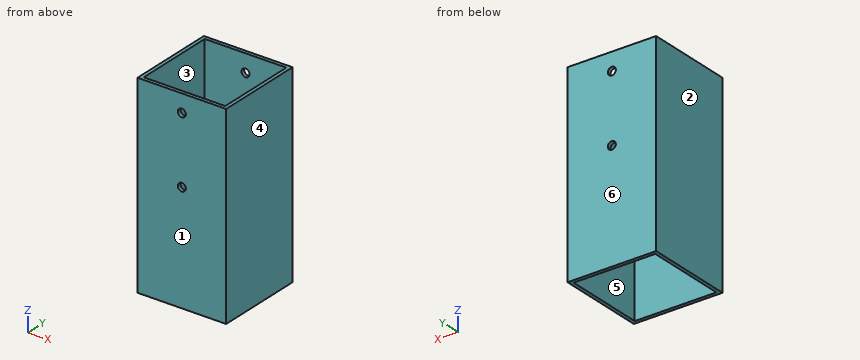
Autodesk Inventor part; units mm, degrees
ref_plane "YZ Plane" through (0, 0, 0) normal (1, 0, 0) x (0, 1, 0)
ref_plane "XZ Plane" through (0, 0, 0) normal (0, 1, 0) x (-1, 0, 0)
ref_plane "XY Plane" through (0, 0, 0) normal (0, 0, 1) x (1, 0, 0)
sketch "スケッチ1" plane through (0, 0, 0) normal (0, 0, 1) x (1, 0, 0)
  line L0 (0, 0) -> (50, 0)
  line L1 (50, 0) -> (50, 50)
  line L2 (50, 50) -> (0, 50)
  line L3 (0, 50) -> (0, 0)
  line L4 (2, 48) -> (48, 48)
  line L5 (48, 48) -> (48, 2)
  line L6 (48, 2) -> (2, 2)
  line L7 (2, 2) -> (2, 48)
  dimension "d0" = 50
  dimension "d1" = 50
  dimension "d2" = 2
extrude "押し出し1" add sketch "スケッチ1" along normal blind 110
sketch "スケッチ5" plane through (0, 50, 0) normal (0, 1, 0) x (1, 0, 0)
  line L0 (50, 0) -> (0, 0)
  line L1 (0, 0) -> (0, -110)
  line L2 (50, -110) -> (0, -110)
  line L3 (50, 0) -> (50, -110)
  line L4 (25, 0) -> (25, -110) construction
  point P0 (0, 0)
  point P1 (25, -62)
  point P2 (25, -100)
  dimension "d42" = 38
  dimension "d43" = 10
hole "穴4" at (25, 50, 62) at (25, 50, 100) direction (0, -1, 0) diameter 4.5 end through all
properties part number "center" material "アルミニウム 6061"
Read the model definition and answer for the solid it produces. Units are mm, in the model's axes. Face numbers are marked on the shaded views. A direction names the side the tool comes from. Coordinates: 2 decimals unless noted, no trailing zeros. Order: outer loops, then holes, each group sorted by start corner. A loop starts at its lowest first (then second) coordinate and runs counter-clockwise, first axis right, second up. Notation, with made-up numbers: M -1,62 L 15,62 A36 ccw 15,98 Z; hole C -10,59 d11. An arc over 180 degrees is marked long. Put each result on its own line as item: value. Start each with the question number.
Item 1: Section C-C, the plane y = 16.5 is taken. Determine the outline of the cut face in (x, z), plus the area to 3 significant figures.
Item 2: For the marked faces 5 and 6, determine the directions among +Z, -Z, +X, -X, +Y, -Y from which every point of the face is accessible in a straight line to the end or side of a thin tool.
Item 3: Section A-A, the plane x = 25 is taken. Determine the outline of the cut face in (y, z).
Item 4: The mould has two halves that part along X. Classify the marked faces 1, 2, 3 and 4: +X half, -X half, draft (parallel to the pull), parting line (faces both ways), or undercut.
Item 5: Section B-B, the plane z = 62 is taken. Determine the outline of the cut face in (x, y).
Item 6: Consider probe 1 along Z at (x, y) = (25, 49.5); probe 2 along X at (y, z) = (46.5, 13). Determine where each line is inside the solid, lowest interval first. Write a range as [from, to].
Computed:
1. outline: M 0,0 L 2,0 L 2,110 L 0,110 Z; M 48,0 L 50,0 L 50,110 L 48,110 Z
1. area: 440 mm2
2. face 5: +Z, -Z
2. face 6: +Z, -Z, +X, -X, +Y
3. outline: M 0,0 L 2,0 L 2,59.75 L 0,59.75 Z; M 0,64.25 L 2,64.25 L 2,97.75 L 0,97.75 Z; M 0,102.25 L 2,102.25 L 2,110 L 0,110 Z; M 48,0 L 50,0 L 50,59.75 L 48,59.75 Z; M 48,64.25 L 50,64.25 L 50,97.75 L 48,97.75 Z; M 48,102.25 L 50,102.25 L 50,110 L 48,110 Z
4. face 1: draft
4. face 2: -X half
4. face 3: undercut
4. face 4: +X half
5. outline: M 0,0 L 22.75,0 L 22.75,2 L 2,2 L 2,48 L 22.75,48 L 22.75,50 L 0,50 Z; M 27.25,0 L 50,0 L 50,50 L 27.25,50 L 27.25,48 L 48,48 L 48,2 L 27.25,2 Z
6. probe 1: z = [0, 59.75], [64.25, 97.75], [102.25, 110]
6. probe 2: x = [0, 2], [48, 50]
